Source: CAD feature listing. Evaluate the final solid. Frame: model axes, mm. Face numbers are marked on the shaded views. Coordinates: 2 decimals unless noted, no trailing zeros. Loops run counter-clockwise (first coordinate to the right, second up) from the corner with the lowest first, then second, coordinate; pieces in that order, holes last. Notation, with made-up numbers: M 57,-34.75 L 87,-34.75 A11 ccw 87,-29.75 Z; hole C 66.5,42.5 d1. An arc over 180 degrees is marked long. Write each question's results on one line, items separated by ' | '. Start each with the question number.
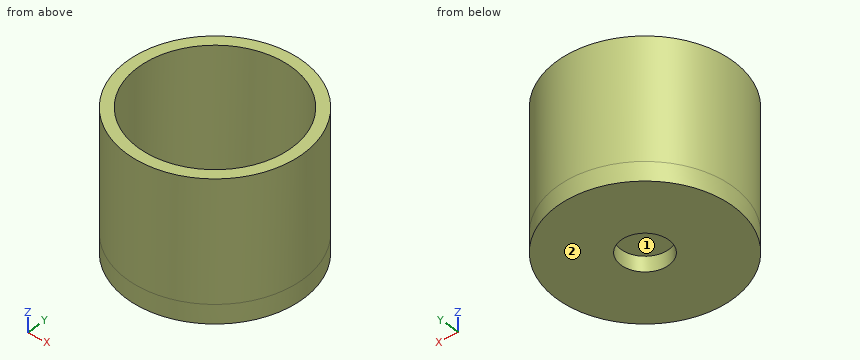
from build123d import *

# Parameters (mm, degrees)
CROQUIS1_R              = 11.6
CROQUIS1_R_2            = 10.1
SALIENTE_EXTRUIR1_DEPTH = 16
SALIENTE_EXTRUIR2_START = 2.5
CROQUIS2_R              = 11.6
SALIENTE_EXTRUIR2_DEPTH = 2.5
CROQUIS3_R              = 3.15
CORTAR_EXTRUIR1_DEPTH   = 2


with BuildPart() as part:
    # Croquis1 → Saliente-Extruir1 (new body)
    with BuildSketch(Plane.XY):
        Circle(CROQUIS1_R)
        Circle(CROQUIS1_R_2, mode=Mode.SUBTRACT)
    extrude(amount=SALIENTE_EXTRUIR1_DEPTH)

    # Croquis2 → Saliente-Extruir2 (add)
    with BuildSketch(Plane(origin=(0, 0, 0), x_dir=(-1, 0, 0), z_dir=(0, 0, -1)).offset(SALIENTE_EXTRUIR2_START)):
        Circle(CROQUIS2_R)
    extrude(amount=-SALIENTE_EXTRUIR2_DEPTH)

    # Croquis3 → Cortar-Extruir1 (cut)
    with BuildSketch(Plane(origin=(0, 0, -2.5), x_dir=(-1, 0, 0), z_dir=(0, 0, -1))):
        Circle(CROQUIS3_R)
    extrude(amount=-CORTAR_EXTRUIR1_DEPTH, mode=Mode.SUBTRACT)


solid = part.part
Item 1: Cut plane B-B (y = 5.75). Output: boundary loops of the cut face in (x, z).
Item 2: First-contact query: pin 1 Ø8 at (x, y) = (0, 0) entering from +Z; pin 2 Ø3 at (x, y) = (-0.5, -0.5) entering from -Z; pin 3 Ø5 at (x, z) = (7, 13.5) entering from +Y. Flat tips, straight axial feed; report the tip coordinate or a pass-through.
Item 3: Line query: probe 1 along Y at (x, z) = (0, 10.75); probe 2 along Y at (x, z) = (0, -1.65); probe 3 along Z at (x, y) = (-3.5, 3). Output: solid intervals per line, ascending.
Item 4: Mould query, pull axis Y, two halves, no side actions, for the marked faces 1 and 2. Classes: +Y half, -Y half, draft (parallel to the pull), parting line (faces both ways), or undercut.
Item 5: Cut plane A-A (x = 0). Output: boundary loops of the cut face in (y, z), then the cut area to 3 significant figures.
Item 6: Cut plane C-C (z = 3.25). Output: boundary loops of the cut face in (x, y), then the cut area to 3 significant figures.
Response values:
1) outline: M -10.07,-2.5 L 10.07,-2.5 L 10.07,16 L 8.3,16 L 8.3,0 L -8.3,0 L -8.3,16 L -10.07,16 Z
2) pin 1: stops at z = 0 | pin 2: stops at z = -0.5 | pin 3: stops at y = 10.69
3) probe 1: y = -11.6 to -10.1, 10.1 to 11.6 | probe 2: y = -11.6 to -3.15, 3.15 to 11.6 | probe 3: z = -2.5 to 0
4) face 1: undercut | face 2: draft
5) outline: M -11.6,-2.5 L -3.15,-2.5 L -3.15,-0.5 L 3.15,-0.5 L 3.15,-2.5 L 11.6,-2.5 L 11.6,16 L 10.1,16 L 10.1,0 L -10.1,0 L -10.1,16 L -11.6,16 Z | area: 93.4 mm2
6) outline: C 0,0 d23.2; hole C 0,0 d20.2 | area: 102 mm2
